Here's the drawing with two shaded views (mm, measured from the low corner). I have some questions. A direction names the side the tool comes from. Coordinates: 2 decimals unless noted, no trailing zeros. Loops run counter-clockwise (first coordinate to the right, second up) from the corner with the lowest first, then second, coordinate; pieces in that order, holes last. Notation, with made-up numbers: (1.25, -18.75) - (34.25, -18.75) arc R33 ccw to (34.25, 10.25) - close; hole circle Ø4 at (84.25, 23.5). An arc over 180 degrees is marked (long way). One line per item, written item: value. Start each with the question number.
(1) If we section it at A-A on y = 20.5: Write out the boundary of the cut face in (x, z), then the cut area to 3 significant figures.
(2) On a 3-axis mill with a long thin cutter (end or side, diameter ignored), from which of +Z, -Z, +X, -X, +Y, -Y can I reach the whole of each face in a straight line? I mean the marked faces 3 and 4. Say none if no direction works.
(3) If we section it at B-B on x = 29.5: Count the separate pieces of the cut face and the enclosed holes in it.
(4) I'm going to push flat-ended pins straight in: P1, Ø1.6, axis at y = 1, z = 15, coming from the +X side; P2, Ø7, axis at y = 32, z = 11, coming from the -X side; P3, Ø1.5, axis at y = 21.5, z = 18, coming from the +X side. Where does each tip first touch, or does it pass through?
(5) If I drill on line 1 along Y through (x, z) = (20, 5.75); line 2 along Y through (x, z) = (43.5, 5.75); line 3 along X through (y, z) = (9, 7), over which ranges is the centre line in solid material (lowest first)? Write a range as from..to.
(6) If we mould it in two halves opening along X, with no side actions, what happens to the marked faces 1 and 2? For each: pulls with the +X half, pulls with the -X half, needs draft (parallel to the pull), parting line crosses it, or undercut.
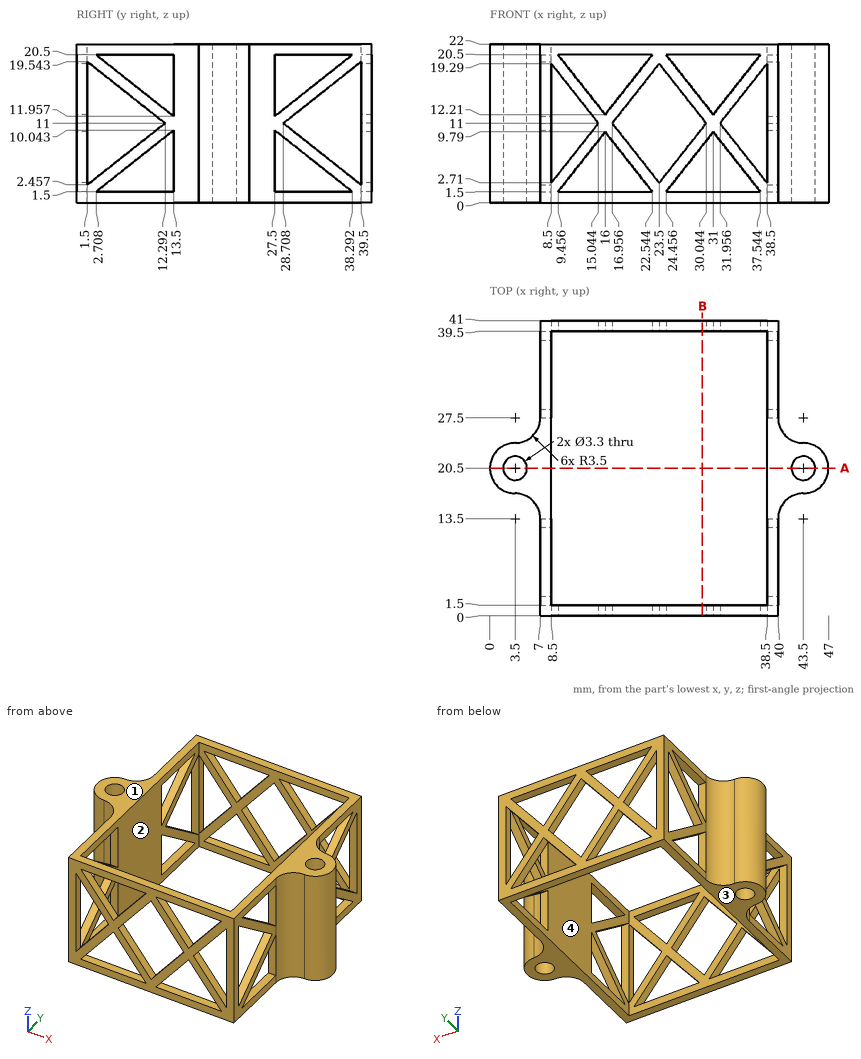
Values:
1. outline: (0, 0) - (1.85, 0) - (1.85, 22) - (0, 22) - close; (5.15, 0) - (8.5, 0) - (8.5, 22) - (5.15, 22) - close; (38.5, 0) - (41.85, 0) - (41.85, 22) - (38.5, 22) - close; (45.15, 0) - (47, 0) - (47, 22) - (45.15, 22) - close
1. area: 229 mm2
2. face 3: -Z, +X, -X, +Y, -Y
2. face 4: +Z, -Z
3. separate pieces: 8
3. enclosed holes: 0
4. P1: stops at x = 40
4. P2: stops at x = 7
4. P3: stops at x = 46.99
5. line 1: y = 0..1.5, 39.5..41
5. line 2: y = 17..18.85, 22.15..24
5. line 3: x = 7..8.5, 38.5..40
6. face 1: needs draft
6. face 2: undercut
